Autodesk Inventor part; units mm, degrees
ref_plane "Work Plane4" through (48.1664, -2.8604, 0) normal (0, 1, 0) x (-1, 0, 0)
ref_plane "Work Plane16" through (-67.2065, -4.4997, 87.6614) normal (0.9396926, 0, 0.3420201) x (0, 1, 0)
ref_plane "Work Plane17" through (60.4164, -7.4791, -11.5) normal (1, 0, 0) x (0, 0, -1)
sketch "Sketch2" plane through (0, 0, 0) normal (0, 0, 1) x (1, 0, 0)
  line L0 (40.7935, -19.9997) -> (-67.2065, -19.9997)
  line L1 (-67.2065, -19.9997) -> (-67.2065, 11.0003)
  circle A0 centre (48.3164, -12.4768) radius 1.575
  arc A1 (44.7809, -16.0123) -> (48.1664, -7.4791) centre (48.3164, -12.4768) ccw
  line L2 (48.1664, 0.0003) -> (48.1664, -7.4791)
  line L3 (48.3164, -12.4768) -> (48.1664, -12.6268)
  line L4 (44.7809, -16.0123) -> (40.7935, -19.9997)
  line L5 (-67.2065, 11.0003) -> (28.1664, 11.0003)
  line L6 (28.1664, 11.0003) -> (48.1664, 0.0003)
  dimension "d19" = 3.15
  dimension "d88" = 10
  dimension "d90" = 0.15
  dimension "d91" = 10.639
  dimension "d111" = 31
  dimension "d135" = 12.4771
  dimension "d176" = 135
  dimension "d177" = 108
extrude "Extrusion1" add sketch "Sketch2" along normal mid plane 23
sketch "Sketch5" plane through (0, 0, 0) normal (0, 0, 1) x (1, 0, 0)
  circle A0 centre (48.3164, -12.4768) radius 1.575
  circle A1 centre (48.3164, -12.4768) radius 5.075
  circle A2 centre (48.3164, -12.4768) radius 1.5
  point P0 (0, 0)
  dimension "d28" = 3
  dimension "d29" = 10.15
extrude "Extrusion3" cut sketch "Sketch5" along normal mid plane 13.41 contours A1
chamfer "Chamfer2" distance 2 angle 45 1 edges at (48.1664, -7.404, 0)
sketch "Sketch15" plane through (48.1664, -7.4791, -11.5) normal (1, 0, 0) x (0, 0, -1)
  arc A0 (-14.3604, 7.4791) -> (-8.6396, 7.4791) centre (-11.5, 7.4791) ccw
  line L0 (-14.3604, 7.4791) -> (-14.3604, 27.4791)
  line L1 (-14.3604, 27.4791) -> (-8.6396, 27.4791)
  line L2 (-8.6396, 27.4791) -> (-8.6396, 7.4791)
  point P0 (-14.3604, 7.4793)
  point P1 (-11.5, 27.4791)
  dimension "d95" = 5.7208
  dimension "d113" = 20
sketch "Sketch19" plane through (-67.2065, -19.9997, 11.5) normal (0, -1, 0) x (1, 0, 0)
  line L0 (63.0729, -6) -> (91.3729, -6)
  line L1 (91.3729, -6) -> (91.3729, -19.5)
  line L2 (91.3729, -19.5) -> (63.0729, -19.5)
  line L3 (63.0729, -19.5) -> (63.0729, -6)
  line L4 (63.0729, -6) -> (91.3729, -19.5) construction
  line L5 (91.3729, -6) -> (63.0729, -19.5) construction
  line L6 (115.3729, -18.205) -> (115.3729, -4.795)
  line L7 (95.3729, 0) -> (0, 0)
  line L8 (108, -23) -> (0, -23)
  circle A0 centre (77.2229, -12.75) radius 8.1325
  point P0 (67.2065, -11.5)
  dimension "d104" = 13.5
  dimension "d114" = 24
  dimension "d195" = 28.3
  dimension "d205" = 6
  dimension "d224" = 16.265
extrude "Extrusion13" cut sketch "Sketch19" against normal blind 30 contours L0 A0 L2 L3 | L0 A0 L2 | L0 L1 L2 A0
sketch "Sketch21" plane through (-67.2065, -19.9997, 11.5) normal (0, -1, 0) x (1, 0, 0)
  line L0 (63.0729, -6) -> (91.3729, -6)
  line L1 (63.0729, -19.5) -> (63.0729, -6) construction
  line L2 (91.3729, -19.5) -> (63.0729, -19.5) construction
  line L3 (63.0729, -6) -> (91.3729, -19.5)
  line L4 (91.3729, -6) -> (63.0729, -19.5)
  line L5 (95.0229, -19.5) -> (59.4229, -19.5)
  line L6 (59.4229, -19.5) -> (59.4229, -6)
  line L7 (59.4229, -6) -> (95.0229, -6)
  line L8 (95.0229, -6) -> (95.0229, -19.5)
  line L9 (95.0229, -19.5) -> (59.4229, -6) construction
  line L10 (59.4229, -19.5) -> (95.0229, -6) construction
  line L11 (108, -23) -> (108, 0)
  point P0 (77.2229, -12.75)
  point P1 (26.7729, -20.5)
  point P2 (26.7729, -7)
  dimension "d164" = 35.6
  dimension "d165" = 13.5
extrude "Extrusion14" cut sketch "Sketch21" against normal blind 10.1
sketch "Sketch20" plane through (-67.2065, 11.0003, 11.5) normal (0, 1, 0) x (1, 0, 0)
  line L0 (115.3729, 23) -> (115.3729, 0)
  line L1 (115.3729, 11.5) -> (95.3729, 11.5)
  point P0 (67.2065, 11.5)
  dimension "d107" = 20
sweep "Sweep3" cut profiles "Sketch15" path "Sketch20" path curves L1
sketch "Sketch22" plane through (48.1664, -7.4791, 11.5) normal (1, 0, 0) x (0, 0, -1)
  circle A0 centre (11.5, -5.0007) radius 1
  line L0 (23, -12.5207) -> (0, -12.5207)
  circle A1 centre (11.5, -9.6079) radius 1
  point P0 (11.5, 7.4791)
  dimension "d126" = 7.52
  dimension "d127" = 2.9128
  dimension "d128" = 2
  dimension "d129" = 2
extrude "Extrusion15" cut sketch "Sketch22" against normal through all
ref_plane "Work Plane4" through (48.1664, -2.8604, 0) normal (0, 1, 0) x (-1, 0, 0)
sketch "Sketch26" plane through (48.1664, -2.8604, 0) normal (0, 1, 0) x (-1, 0, 0)
  line L0 (0, -6.705) -> (0, 6.705)
  arc A0 (16.24, -0.7321) -> (16.24, 0.7321) centre (16.24, 0) ccw
  line L1 (16.24, -0.7321) -> (0, -0.7321)
  line L2 (16.24, 0.7321) -> (0, 0.7321)
  line L3 (0, 0.7321) -> (0, -0.7321)
  point P0 (48.1664, 0)
  dimension "d147" = 1.4642
chamfer "Chamfer3" distance 3.6 angle 45 1 edges at (44.7278, -16.0654, 0)
extrude "Extrusion22" add sketch "Sketch26" along normal up to surface surface through (48.1664, 0.0003, 0) normal (0.4819187, 0.8762159, 0)
sketch "Sketch29" plane through (-67.2065, -9.8997, 11.5) normal (0, -1, 0) x (1, 0, 0)
  line L0 (95.0229, -6) -> (95.0229, -19.5)
  line L1 (91.3729, -15.7347) -> (95.0229, -15.7347)
  line L2 (95.0229, -15.7347) -> (95.0229, -9.7653)
  line L3 (95.0229, -9.7653) -> (91.3729, -9.7653)
  line L4 (91.3729, -9.7653) -> (91.3729, -15.7347)
  line L5 (91.3729, -19.5) -> (91.3729, -15.7347)
  line L6 (91.3729, -9.7653) -> (91.3729, -6)
  point P0 (67.2065, -11.5)
  dimension "d202" = 3.7653
  dimension "d203" = 3.7653
extrude "Extrusion23" cut sketch "Sketch29" against normal through all
pattern_linear "Rectangular Pattern6" count 2 spacing -31.95 along (1, 0, 0) of "Extrusion23"
pattern_linear "Rectangular Pattern8" count 4 spacing 30 along (0, 0, 1) of "Extrusion1", "Extrusion3", "Chamfer2", "Sweep3", "Extrusion15", "Chamfer3", "Extrusion22"
sketch "Sketch30" plane through (0, 0, 11.5) normal (0, 0, 1) x (1, 0, 0)
  line L0 (48.1664, -7.4791) -> (48.1664, 0.0003)
  line L1 (48.1664, 0.0003) -> (28.1664, 11.0003)
  line L2 (28.1664, 11.0003) -> (-67.2065, 11.0003)
  line L3 (-67.2065, 11.0003) -> (-67.2065, -19.9997)
  line L4 (-67.2065, -19.9997) -> (40.7935, -19.9997)
  line L5 (40.7935, -19.9997) -> (44.7809, -16.0123)
  arc A0 (44.7809, -16.0123) -> (48.1664, -7.4791) centre (48.3164, -12.4768) ccw
  circle A1 centre (48.3164, -12.4768) radius 1.575
  circle A2 centre (48.3164, -12.4768) radius 5
  point P0 (0, 0)
  point P1 (28.1664, -19.9997)
extrude "Extrusion24" add sketch "Sketch30" along normal up to surface (7 mm away) contours A2 L5 L4 L3 L2 L1 L0
pattern_linear "Rectangular Pattern9" count 3 spacing 30 along (0, 0, 1) of "Extrusion24"
pattern_linear "Rectangular Pattern10" count 6 spacing 18.5 along (0, 0, 1) of "Extrusion13", "Extrusion14", "Extrusion23", "Rectangular Pattern6"
sketch "Sketch32" plane through (-67.2065, -19.9997, -11.5) normal (0, -1, 0) x (1, 0, 0)
  line L0 (43.9229, 7) -> (57.4229, 7)
  line L1 (57.4229, 7) -> (57.4229, 35.3)
  line L2 (57.4229, 35.3) -> (43.9229, 35.3)
  line L3 (43.9229, 35.3) -> (43.9229, 7)
  line L4 (57.4229, 35.3) -> (43.9229, 7)
  line L5 (57.4229, 7) -> (43.9229, 35.3)
  line L6 (59.4229, 3.5) -> (59.4229, 17)
  line L7 (108, 0) -> (0, 0)
  point P0 (67.2065, 11.5)
  dimension "d218" = 28.3
  dimension "d219" = 13.5
  dimension "d225" = 2
  dimension "d226" = 7
extrude "Extrusion26" cut sketch "Sketch32" against normal blind 30
sketch "Sketch33" plane through (-67.2065, -19.9997, -11.5) normal (0, -1, 0) x (1, 0, 0)
  line L0 (43.9229, 35.3) -> (57.4229, 35.3)
  line L1 (57.4229, 35.3) -> (57.4229, 7)
  line L2 (57.4229, 7) -> (43.9229, 7)
  line L3 (43.9229, 7) -> (43.9229, 35.3)
  line L4 (57.4229, 35.3) -> (43.9229, 7)
  line L5 (57.4229, 7) -> (43.9229, 35.3)
  line L6 (57.4229, 3.35) -> (43.9229, 3.35)
  line L7 (43.9229, 3.35) -> (43.9229, 38.95)
  line L8 (43.9229, 38.95) -> (57.4229, 38.95)
  line L9 (57.4229, 38.95) -> (57.4229, 3.35)
  line L10 (57.4229, 3.35) -> (43.9229, 38.95) construction
  line L11 (43.9229, 3.35) -> (57.4229, 38.95) construction
  point P0 (67.2065, 11.5)
  point P1 (50.6729, 21.15)
  point P2 (57.4229, 7)
  dimension "d240" = 13.5
  dimension "d241" = 35.6
extrude "Extrusion27" cut sketch "Sketch33" against normal blind 10.1
sketch "Sketch34" plane through (-67.2065, -9.8997, -11.5) normal (0, -1, 0) x (1, 0, 0)
  line L0 (57.4229, 3.35) -> (43.9229, 3.35)
  line L1 (43.9229, 7) -> (57.4229, 7)
  line L2 (57.4229, 7) -> (43.9229, 7)
  line L3 (53.6579, 7) -> (47.6879, 7)
  line L4 (47.6879, 7) -> (47.6879, 3.35)
  line L5 (47.6879, 3.35) -> (53.6579, 3.35)
  line L6 (53.6579, 3.35) -> (53.6579, 7)
  line L7 (57.4229, 35.3) -> (57.4229, 7)
  line L8 (57.4229, 7) -> (53.6579, 7)
  line L9 (47.6879, 7) -> (43.9229, 7)
  point P0 (67.2065, 11.5)
  point P1 (53.6579, 3.35)
  point P2 (47.6879, 7)
  dimension "d242" = 3.765
extrude "Extrusion28" cut sketch "Sketch34" against normal through all
pattern_linear "Rectangular Pattern11" count 2 spacing 31.95 along (0, 0, 1) of "Extrusion28"
pattern_linear "Rectangular Pattern12" count 2 spacing 70.5 along (0, 0, 1) of "Extrusion26", "Extrusion27", "Extrusion28", "Rectangular Pattern11"
ref_plane "Work Plane16" through (-67.2065, -4.4997, 87.6614) normal (0.9396926, 0, 0.3420201) x (0, 1, 0)
sketch "Sketch37" plane through (-67.2065, -4.4997, 87.6614) normal (0.9396926, 0, 0.3420201) x (0, 1, 0)
  line L0 (-15.5, -7.5229) -> (-7.9771, 0)
  circle A0 centre (-7.9771, 0.15) radius 4.925
  circle A1 centre (-7.9771, 0.15) radius 1.575
  point P0 (4.4997, -105.3608)
  dimension "d271" = 0.15
  dimension "d272" = 9.85
  dimension "d273" = 3.15
sketch "Sketch39" plane through (-67.2065, -19.9997, 101.5) normal (0, 0, 1) x (1, 0, 0)
  line L0 (95.3729, 31) -> (0, 31)
  line L1 (95.3729, 0) -> (0, 0)
  line L2 (0, 31) -> (0, 0)
  line L3 (30.3, 0) -> (7, 0)
  line L4 (7, 0) -> (7, 31)
  line L5 (7, 31) -> (30.3, 31)
  line L6 (30.3, 31) -> (30.3, 0)
  point P0 (67.2065, 19.9997)
  point P1 (30.3, 31)
  point P2 (7, 0)
  dimension "d275" = 23.3
  dimension "d276" = 7
extrude "Extrusion36" cut sketch "Sketch39" against normal blind 41 contours L6 L1 L4 L0
sketch "Sketch40" plane through (-36.9065, -19.9997, 101.5) normal (-1, 0, 0) x (0, 0, 1)
  line L0 (-41, 31) -> (-41, 0)
  line L1 (-41, 15.5) -> (-26, 15.5)
  circle A0 centre (-26, 15.5) radius 15
  circle A1 centre (-26, 15.5) radius 1.575
  point P0 (-101.5, 19.9997)
  dimension "d279" = 15
  dimension "d280" = 30
  dimension "d281" = 3.15
extrude "Extrusion37" cut sketch "Sketch40" along normal through all contours A1
extrude "Extrusion38" cut sketch "Sketch40" against normal blind 10 contours A1
chamfer "Chamfer5" distance 13.75 angle 45 1 edges at (-36.9065, -4.4997, 101.5)
ref_plane "Work Plane17" through (60.4164, -7.4791, -11.5) normal (1, 0, 0) x (0, 0, -1)
sketch "Sketch41" plane through (60.4164, -7.4791, -11.5) normal (1, 0, 0) x (0, 0, -1)
  line L0 (-0.6, -10.9819) -> (-22.4, -10.9819)
  line L1 (-22.4, -10.9819) -> (-22.4, 3.5681)
  line L2 (-22.4, 3.5681) -> (-0.6, 3.5681)
  line L3 (-0.6, 3.5681) -> (-0.6, -10.9819)
  line L4 (0, -9.9977) -> (0, 0.0023)
  line L5 (-18.205, -11.1319) -> (-4.795, -11.1319)
  line L6 (-23, 0.0023) -> (-23, -9.9977)
  point P0 (-11.5, 7.4791)
  point P1 (0, 0)
  point P2 (0, -8.5333)
  point P3 (-23, -8.5333)
  point P4 (-23, 0)
  dimension "d293" = 14.55
  dimension "d306" = 0.15
  dimension "d307" = 0.6
  dimension "d308" = 0.6
  dimension "d311" = 21.8
extrude "Extrusion39" cut sketch "Sketch41" against normal blind 31.1 keep common part
sketch "Sketch42" plane through (-67.2065, -19.9997, -11.5) normal (0, -1, 0) x (1, 0, 0)
  circle A0 centre (103.7729, 4.1009) radius 1.575
  line L0 (103.7729, 11.5) -> (97.0263, 11.5)
  circle A1 centre (103.7729, 18.8991) radius 1.575
  point P0 (67.2065, 11.5)
  dimension "d302" = 3.15
  dimension "d303" = 0
  dimension "d309" = 3.15
  dimension "d310" = 7.3991
extrude "Extrusion40" cut sketch "Sketch42" against normal blind 25
ref_plane "Work Plane11" through (48.1664, -2.8604, 30) normal (0, 1, 0) x (-1, 0, 0)
ref_plane "Work Plane12" through (48.1664, -2.8604, 60) normal (0, 1, 0) x (-1, 0, 0)
ref_plane "Work Plane13" through (48.1664, -2.8604, 90) normal (0, 1, 0) x (-1, 0, 0)
equation "\"d88\" = diametroFueraUnion"
equation "\"d90\" = tolerancia"
equation "\"d28\" = diametroDentroUnion"
equation "\"d29\" = diametroFueraUnion + tolerancia"
equation "\"d10\" = 10.639"
equation "\"d16\" = 135deg"
equation "\"d26\" = 135deg"
equation "\"d27\" = 135deg"
equation "\"d30\" = 135deg"
equation "\"d34\" = 23"
equation "\"d35\" = 0"
equation "\"d40\" = 135deg"
equation "\"d41\" = 10.639"
equation "\"d42\" = 11.8875"
equation "\"d43\" = 0"
equation "\"diametroDentroUnion\" = 3"
equation "\"diametroFueraUnion\" = 10"
equation "\"d45\" = 15"
equation "\"d39\" = diametroDentroUnion"
equation "\"anchoServo\" = 12.2"
equation "\"tolerancia\" = 0.15"
equation "\"d193\" = 0.15"
equation "\"d199\" = 0.15"
equation "\"d215\" = 0.15"
equation "\"d216\" = 0.15"
equation "\"servoLargo\" = 28"
equation "\"servoLargoConOrejas\" = 35.3"
equation "\"servoAncho\" = 13.2"
equation "\"ServoAlto\" = 29.7"
equation "\"diametroPolea\" = 16.265"
properties part number "sujeciones_dedos_V13"
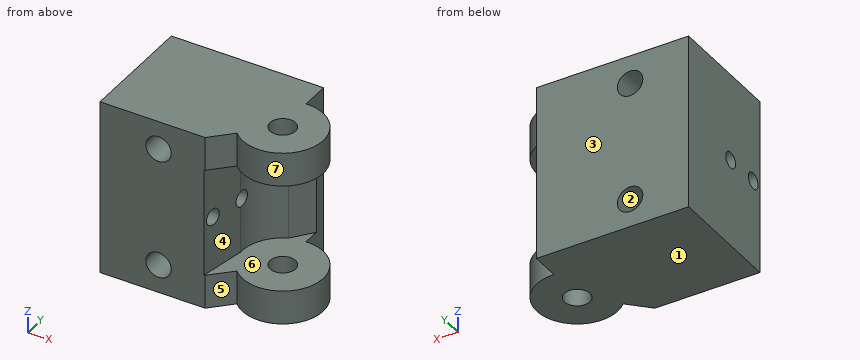
Here's how the part is built. I have some questions about the finished solid (model axes, mm). Face numbers are marked on the shaded views. A direction names the side the tool comes from. Coordinates: 2 decimals unless noted, no trailing zeros. Loops run counter-clockwise (first coordinate to the right, second up) from the corner with the lowest first, then second, coordinate; pieces in that order, holes last. Notation, with made-up numbers: (39, 57) - (68, 57) arc R19 ccw to (68, 85) - close; hole circle Ø1 at (-29, 17). An arc over 180 degrees is marked (long way). Answer as CSV lines item,"result".
Q1. We'd pull the mould along Z, two halves only. Please class the marked faces 1, 2, 3 and 4: pulls with the +Z half, pulls with the -Z half, needs draft (parallel to the pull), parting line crosses it, or undercut.
Response:
face 1,"pulls with the -Z half"
face 2,"undercut"
face 3,"needs draft"
face 4,"undercut"
Q2. If we section it at D-D, the plane x = 51.75: Write out the boundary of the cut face in (y, z) (3 decimals).
Response:
outline,"(-16.111, -10.9) - (-8.842, -10.9) - (-8.842, -6.705) - (-16.111, -6.705) - close; (-16.111, 6.705) - (-8.842, 6.705) - (-8.842, 10.9) - (-16.111, 10.9) - close"
Q3. For pin 1 (3 mm diameter, centred on y = -17.087, z = 0, fed in from +X); pin 2 (4 mm diameter, centred on x = 36.57, z = -7.4, fed in from +Y); pin 3 (1.1 mm diameter, centred on y = -5.5, z = 1, fed in from +X), each with a flat end and sliding along its axis, tell me the tip position at first contact or that it passes through.
Response:
pin 1,"x = 42.74"
pin 2,"y = -3.91"
pin 3,"x = 48.17"
Q4. If we section it at B-B, the plane z = 0: Write out the boundary of the cut face in (x, y) (3 decimals), and give its area (3 significant figures).
Response:
outline,"(29.316, -18.461) - (42.21, -18.461) - (42.278, -18.087) - (29.316, -18.087) - close; (29.316, -16.087) - (42.645, -16.087) - (43.123, -13.48) - (29.316, -13.48) - close; (29.316, -11.48) - (43.34, -11.48) arc R5.075 cw to (46.218, -7.856) - (48.166, -5.404) - (48.166, -3.911) - (29.316, -3.911) - close"
area,"166 mm2"
Q5. If we section it at C-C, the plane z = -7.75: Write out the boundary of the cut face in (x, y) (3 decimals).
Response:
outline,"(29.316, -18.461) - (35.031, -18.461) - (35.031, -3.911) - (29.316, -3.911) - close; (38.102, -18.461) - (42.332, -18.461) - (44.781, -16.012) arc R5 ccw (long way) to (48.166, -7.479) - (48.166, -3.911) - (38.102, -3.911) - close; hole circle Ø3.15 at (48.316, -12.477)"
Q6. For the marked faces 5, 6 and 7, which set-ups out of +Z, -Z, +X, -X, +Y, -Y let a thin tool reach every point of the face, with its end or its side?
Response:
face 5,"+Z, -Z, -Y"
face 6,"+X, -Y"
face 7,"+Z, -Z"
Q7. If we section it at A-A, the plane x = 37.75: Write out the boundary of the cut face in (y, z), and give its area (3 significant figures).
Response:
outline,"(-18.46, -10.9) - (-3.91, -10.9) - (-3.91, -8.44) - (-18.46, -8.44) - close; (-18.46, -6.36) - (-3.91, -6.36) - (-3.91, 6.36) - (-18.46, 6.36) - close; (-18.46, 8.44) - (-3.91, 8.44) - (-3.91, 10.9) - (-18.46, 10.9) - close; hole circle Ø2 at (-17.09, 0); hole circle Ø2 at (-12.48, 0)"
area,"250 mm2"
Q8. If I drill on L1, parallel to Y at x = 33.5, z = 0; L2, parallel to Z at x = 50, y = -17 (3 decimals); L3, parallel to X at y = -11.75, z = -7, over which ranges is the centre line in solid material (lowest first)? Write a range as [from, to].
Response:
L1,"[-18.46, -18.09], [-16.09, -13.48], [-11.48, -3.91]"
L2,"[-10.9, -6.705], [6.705, 10.9]"
L3,"[29.32, 35.04], [38.09, 46.92], [49.71, 53.26]"
